Can you work these out from the model? Positions are in its coordinate system, mm. Coordinates: 2 decimals unless noted, no trailing zeros. Order: outer loops, then holes, each group sorted by start corner. A loop starts at its lowest first (then second) coordinate and runs counter-clockwise, first axis right, second up.
```python
from build123d import *

# Parameters (mm, degrees)
SKETCH1_W           = 300
SKETCH1_H           = 500
BOSS_EXTRUDE1_DEPTH = 1200
SKETCH2_R           = 3
BOSS_EXTRUDE2_DEPTH = 28


with BuildPart() as part:
    # Sketch1 → Boss-Extrude1 (new body)
    with BuildSketch(Plane.XY):
        with Locations((66.901408451, -71.830985915)):
            Rectangle(SKETCH1_W, SKETCH1_H)
    extrude(amount=BOSS_EXTRUDE1_DEPTH)

    # Sketch2 → Boss-Extrude2 (add)
    with BuildSketch(Plane(origin=(0, 178.169014085, 0), x_dir=(1, 0, 0), z_dir=(0, 1, 0))):
        with Locations(Location((66.901408451, -100, 0), (0, 0, 90))):
            Circle(SKETCH2_R)
        with Locations(Location((66.901408451, -300, 0), (0, 0, 90))):
            Circle(SKETCH2_R)
        with Locations(Location((66.901408451, -500, 0), (0, 0, 90))):
            Circle(SKETCH2_R)
        with Locations(Location((66.901408451, -700, 0), (0, 0, 90))):
            Circle(SKETCH2_R)
        with Locations(Location((66.901408451, -900, 0), (0, 0, 90))):
            Circle(SKETCH2_R)
        with Locations(Location((66.901408451, -1100, 0), (0, 0, 90))):
            Circle(SKETCH2_R)
    extrude(amount=BOSS_EXTRUDE2_DEPTH)


solid = part.part
```
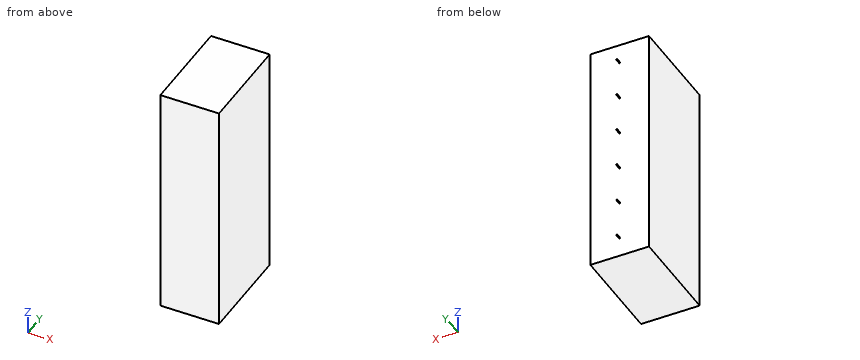
1. I'm going to push flat-ended pins straight in: pin 1 (12 mm diameter, centred on x = -15, y = -151.5, fed in from -Z); pin 2 (2 mm diameter, centred on x = 186, z = 972, fed in from +Y). Where does each tip first touch, or does it pass through?
Completed:
pin 1: stops at z = 0
pin 2: stops at y = 178.17
2. Imagine slicing it at B-B on z = 1048.5. Please give me the cut outline in (x, y).
Completed:
outline: (-83.1, -321.83) - (216.9, -321.83) - (216.9, 178.17) - (-83.1, 178.17) - close
3. Please list where this line runs through material, in increasing order: probe 1 along Y at (x, z) = (-52.5, 570).
Completed:
probe 1: y = -321.83 to 178.17
4. Imagine slicing it at A-A on x = 91. Please give me the cut outline in (y, z), then the cut area to 3 significant figures.
Completed:
outline: (-321.83, 0) - (178.17, 0) - (178.17, 1200) - (-321.83, 1200) - close
area: 600,000 mm2
